```python
from build123d import *

# Parameters (mm, degrees)
BOSS_EXTRUDE1_DEPTH      = 160
BOSS_EXTRUDE1_DEPTH_BACK = 5
SKETCH1_R                = 7.75
SKETCH1_R_2              = 7
SKETCH5_R                = 7.5
BOSS_EXTRUDE3_DEPTH      = 72.0622032
SKETCH7_R                = 7.75
SKETCH7_R_2              = 7
BOSS_EXTRUDE5_DEPTH      = 25


with BuildPart() as part:
    # Sketch1 → Boss-Extrude1 (new, two sides: drawn at the far end of the back side and taken through both)
    with BuildSketch(Plane(origin=(0, 0, 0), x_dir=(1, 0, 0), z_dir=(0, 1, 0)).offset(-BOSS_EXTRUDE1_DEPTH_BACK)):
        with Locations(Location((0, 0, 0), (0, 0, 270))):
            Circle(SKETCH1_R)
        with Locations(Location((0, 0, 0), (0, 0, 270))):
            Circle(SKETCH1_R_2, mode=Mode.SUBTRACT)
    extrude(amount=BOSS_EXTRUDE1_DEPTH + BOSS_EXTRUDE1_DEPTH_BACK)

    # Sketch5 → Boss-Extrude3 (add)
    with BuildSketch(Plane(origin=(0, 0, 0), x_dir=(0, 0, -1), z_dir=(1, 0, 0))):
        with Locations(Location((0, 75, 0), (0, 0, 180))):
            Circle(SKETCH5_R)
    extrude(amount=BOSS_EXTRUDE3_DEPTH)

    # Sketch7 → Boss-Extrude5 (add)
    with BuildSketch(Plane(origin=(0, 160, 0), x_dir=(1, 0, 0), z_dir=(0, 1, 0))):
        with Locations(Location((0, 0, 0), (0, 0, 270))):
            Circle(SKETCH7_R)
        with Locations(Location((0, 0, 0), (0, 0, 270))):
            Circle(SKETCH7_R_2, mode=Mode.SUBTRACT)
    extrude(amount=BOSS_EXTRUDE5_DEPTH)


solid = part.part
```
Geometry: final body of the model. Coordinates: model frame, mm. A direction names the side the tool comes from. Give positions to 0.01 mm unless a question says otherwise; leave off trailing zeros. Loops run counter-clockwise (first coordinate to the right, second up) from the corner with the lowest first, then second, coordinate; pieces in that order, holes last. Notation, with made-up numbers: (25, -11.5) -> (60, -11.5) arc R23 ccw to (60, -0.5) -> close; hole circle Ø2 at (-38, 59.5). An arc over 180 degrees is marked (long way). Use CSV: the item, a comma, the result in double quotes.
(1) Cut plane B-B (y = 75). Output: boundary loops of the cut face in (x, z).
From the geometry:
outline,"(1.95, -7.5) -> (72.06, -7.5) -> (72.06, 7.5) -> (1.95, 7.5) arc R7.75 ccw (long way) to start; hole (0, -7) -> (0, 7) arc R7 ccw to start"
(2) First-contact query: P1, Ø3, axis at x = 51.5, z = -5.5, coming from the +Y side; P2, Ø2, axis at y = 127, z = -4, coming from the +X side; P3, Ø6, axis at y = 51.5, z = -6, coming from the -X side. Flat tips, straight axial feed; report the tip coordinate or a pass-through.
From the geometry:
P1,"y = 81.34"
P2,"x = 7.15"
P3,"x = -7.15"
(3) Cut plane C-C (x = 9.5). Output: boundary loops of the cut face in (y, z).
From the geometry:
outline,"circle Ø15 at (75, 0)"
(4) Cut plane D-D (y = 24.5). Output: boundary loops of the cut face in (x, z), plus the area to 3 significant figures.
From the geometry:
outline,"circle Ø15.5 at (0, 0); hole circle Ø14 at (0, 0)"
area,"34.8 mm^2"
(5) Ray query, line 1 along X through (y, z) = (86, 0); line 2 along X through (y, z) = (96, 4.5); line 3 along Z through (x, y) = (48.5, 75). Return the intervals inside material, ascending. Write a range as [from, to].
From the geometry:
line 1,"[-7.75, -7], [7, 7.75]"
line 2,"[-6.31, -5.36], [5.36, 6.31]"
line 3,"[-7.5, 7.5]"
(6) Access query for faces 1 (the face through (-4, -5, -6)), 2 (the face through (36.516, 81.654, 3.461)), 3 (the face through (-6.834, 88.67, -1.517)). Directions: +Z, -Z, +X, -X, +Y, -Y. A direction counts if a zero-diameter tool reaches every point of the face in a straight line with its end or side. Return the directions, or none.
From the geometry:
face 1,"+Z, -Z, +X, -X, -Y"
face 2,"+X"
face 3,"none"
(7) Pull-direction query (Z, two-part tool) for faces 4 (the face through (0, 75, 0)), 5 (the face through (7.684, 88.67, -1.009)), 6 (the face through (-4, 185, -6)); classes: released by +Z, released by -Z, zero draft, split by the parting line, or undercut.
From the geometry:
face 4,"undercut"
face 5,"split by the parting line"
face 6,"zero draft"
(8) Cut plane A-A (z = 0). Output: boundary loops of the cut face in (x, y).
From the geometry:
outline,"(-7.75, -5) -> (-7, -5) -> (-7, 185) -> (-7.75, 185) -> close; (0, 67.5) -> (7, 67.5) -> (7, -5) -> (7.75, -5) -> (7.75, 67.5) -> (72.06, 67.5) -> (72.06, 82.5) -> (7.75, 82.5) -> (7.75, 185) -> (7, 185) -> (7, 82.5) -> (0, 82.5) -> close"
